```python
from build123d import *

# Parameters (mm, degrees)
F0_W     = 5
F0_H     = 11
F1_DEPTH = 4
F0_W_2   = 15
F0_H_2   = 23
F0_R     = 2
F0_R_2   = 0.5
F2_DEPTH = 1.5


with BuildPart() as f1:
    # F0 (on Top) → F1 (new body)
    with BuildSketch(Plane.XY):
        Polygon((-1.5, -10.573518), (4.5, -10.573518), (4.5, 10.573518), (-1.5, 10.573518), (-1.5, 5.5), (-1.5, -5.5), align=None)
        with Locations((-4, 0)):
            Rectangle(F0_W, F0_H)
    extrude(amount=F1_DEPTH)

    # F0 (on Top) → F2 (join)
    with BuildSketch(Plane.XY):
        Rectangle(F0_W_2, F0_H_2)
        with Locations((-4.5, -8.5)):
            Circle(F0_R, mode=Mode.SUBTRACT)
        with Locations((6, -10.5)):
            Circle(F0_R_2, mode=Mode.SUBTRACT)
        with Locations((6, -7.5)):
            Circle(F0_R_2, mode=Mode.SUBTRACT)
        with Locations((6, -4.5)):
            Circle(F0_R_2, mode=Mode.SUBTRACT)
        with Locations((6, -1.5)):
            Circle(F0_R_2, mode=Mode.SUBTRACT)
        Polygon((4.5, 10.573518), (4.5, -10.573518), (-1.5, -10.573518), (-1.5, -5.5), (-6.5, -5.5), (-6.5, 5.5), (-1.5, 5.5), (-1.5, 10.573518), align=None, mode=Mode.SUBTRACT)
        with Locations((-4.5, 8.5)):
            Circle(F0_R, mode=Mode.SUBTRACT)
        with Locations((6, 1.5)):
            Circle(F0_R_2, mode=Mode.SUBTRACT)
        with Locations((6, 4.5)):
            Circle(F0_R_2, mode=Mode.SUBTRACT)
        with Locations((6, 7.5)):
            Circle(F0_R_2, mode=Mode.SUBTRACT)
        with Locations((6, 10.5)):
            Circle(F0_R_2, mode=Mode.SUBTRACT)
    extrude(amount=F2_DEPTH)


solid = f1.part
```
Input: part model. Units: mm. Frame: model coordinates. A direction names the side the tool comes from. Give positions to 0.01 mm unless a question says otherwise; leave off trailing zeros. Order: outer loops, then holes, each group sorted by start corner. A loop starts at its lowest first (then second) coordinate and runs counter-clockwise, first axis right, second up. Notation, with made-up numbers: M 45.5,58 L 104.5,58 A10 cw 104.5,65 Z; hole C 85,-28 d7. An arc over 180 degrees is marked long. Return JSON: item names as keys, results as strings.
1) Access query for faces 4 (the face through (-1.5, -8, 3)), 5 (the face through (-4, 5.5, 3)), 6 (the face through (1, -10.574, 3)), 7 (the face through (-6.5, 0, 3)). Directions: +Z, -Z, +X, -X, +Y, -Y. A direction counts if a zero-diameter tool reaches every point of the face in a straight line with its end or side. Return the directions, or none.
Taken from the geometry:
{"face 4": "+Z, -X, -Y", "face 5": "+Z, -X, +Y", "face 6": "+Z, +X, -X, -Y", "face 7": "+Z, -X, +Y, -Y"}
2) Line query: L1, parallel to Z at x = 7, y = 6.5; L2, parallel to Y at x = 1.75, z = 2.05; L3, parallel to Y at x = -1.75, z = 2.4. Output: solid intervals per line, ascending. Write a range as [from, to].
Taken from the geometry:
{"L1": "z = [0, 1.5]", "L2": "y = [-10.57, 10.57]", "L3": "y = [-5.5, 5.5]"}
3) Section query B-B on y = 8.5. Output: boundary loops of the cut face in (x, z).
Taken from the geometry:
{"outline": "M -7.5,0 L -6.5,0 L -6.5,1.5 L -7.5,1.5 Z; M -2.5,0 L 7.5,0 L 7.5,1.5 L 4.5,1.5 L 4.5,4 L -1.5,4 L -1.5,1.5 L -2.5,1.5 Z"}
4) Section query C-C on z = 1. Count the separate pieces of the cut face and the enclosed holes in it, and give its area (3 significant figures).
Taken from the geometry:
{"separate pieces": "1", "enclosed holes": "10", "area": "314 mm2"}
5) Contact query for flat-ended pins moving along their axis: pin 1 (1 mm diameter, centred on x = 3, z = 3, fed in from +Y); pin 2 (0.8 mm diameter, centred on y = 8, z = 3, fed in from -X); pin 3 (0.8 mm diameter, centred on y = 0, z = 2.5, fed in from -X). Output: stop coordinate, or through.
Taken from the geometry:
{"pin 1": "stops at y = 10.57", "pin 2": "stops at x = -1.5", "pin 3": "stops at x = -6.5"}
6) Section query D-D on y = 4.5. Output: boundary loops of the cut face in (x, z).
Taken from the geometry:
{"outline": "M -7.5,0 L 5.5,0 L 5.5,1.5 L 4.5,1.5 L 4.5,4 L -6.5,4 L -6.5,1.5 L -7.5,1.5 Z; M 6.5,0 L 7.5,0 L 7.5,1.5 L 6.5,1.5 Z"}
7) Section query A-A on x = -4.5. Output: boundary loops of the cut face in (y, z).
Taken from the geometry:
{"outline": "M -11.5,0 L -10.5,0 L -10.5,1.5 L -11.5,1.5 Z; M -6.5,0 L 6.5,0 L 6.5,1.5 L 5.5,1.5 L 5.5,4 L -5.5,4 L -5.5,1.5 L -6.5,1.5 Z; M 10.5,0 L 11.5,0 L 11.5,1.5 L 10.5,1.5 Z"}
8) Mould query, pull axis X, two halves, no side actions, for faces 1 (the face through (-4.76, 10.483, 0.74)), 2 (the face through (0, 11.5, 1)), 3 (the face through (4.5, 0, 3)). Classes: released by +X, released by -X, zero draft, split by the parting line, or undercut.
Taken from the geometry:
{"face 1": "undercut", "face 2": "zero draft", "face 3": "released by +X"}
